```python
from build123d import *

# Parameters (mm, degrees)
BOSS_EXTRUDE1_DEPTH  = 6
CUT_EXTRUDE15_DEPTH  = 103.528044944
SKETCH19_OUTSIDE_W   = 185.536
SKETCH19_OUTSIDE_H   = 176.439
SKETCH19_OUTSIDE_W_2 = 80
SKETCH19_OUTSIDE_H_2 = 40
CUT_EXTRUDE16_DEPTH  = 103.528044944
SKETCH20_R           = 2.4
CUT_EXTRUDE17_DEPTH  = 84.234608187


with BuildPart() as part:
    # Sketch1 → Boss-Extrude1 (new, symmetric)
    with BuildSketch(Plane(origin=(0, 0, 0), x_dir=(1, 0, 0), z_dir=(0, 1, 0))):
        with BuildLine():
            ThreePointArc((36.224522061, -62.223661106), (0, 72), (-36.224522061, -62.223661106))
            ThreePointArc((-36.224522061, -62.223661106), (-32.797800029, -62.818856853), (-29.811944095, -61.035223988))
            ThreePointArc((-29.811944095, -61.035223988), (0, -46.75), (29.811944095, -61.035223988))
            ThreePointArc((29.811944095, -61.035223988), (32.797800029, -62.818856853), (36.224522061, -62.223661106))
        make_face()
    extrude(amount=BOSS_EXTRUDE1_DEPTH, both=True)

    # Sketch17 → Cut-Extrude15 (cut, through all)
    with BuildSketch(Plane(origin=(0, 6, 0), x_dir=(1, 0, 0), z_dir=(0, 1, 0))):
        with BuildLine():
            Line((11.501290376, 48.2), (-11.501290376, 48.2))
            ThreePointArc((-11.501290376, 48.2), (-13.503335986, 55.621683574), (-18.824890953, 61.168811339))
            ThreePointArc((-18.824890953, 61.168811339), (-13.394450398, 62.582654933), (-7.861037919, 63.515384615))
            ThreePointArc((-7.861037919, 63.515384615), (0, 57), (7.861037919, 63.515384615))
            ThreePointArc((7.861037919, 63.515384615), (13.394450398, 62.582654933), (18.824890953, 61.168811339))
            ThreePointArc((18.824890953, 61.168811339), (13.503335986, 55.621683574), (11.501290376, 48.2))
        make_face()
    extrude(amount=-CUT_EXTRUDE15_DEPTH, mode=Mode.SUBTRACT)

    # Sketch19 outside → Cut-Extrude16 (cut, through all)
    with BuildSketch(Plane(origin=(0, 6, 0), x_dir=(1, 0, 0), z_dir=(0, 1, 0))):
        with Locations((0, 4.5485)):
            Rectangle(SKETCH19_OUTSIDE_W, SKETCH19_OUTSIDE_H)
        with Locations((0, 57)):
            Rectangle(SKETCH19_OUTSIDE_W_2, SKETCH19_OUTSIDE_H_2, mode=Mode.SUBTRACT)
    extrude(amount=-CUT_EXTRUDE16_DEPTH, mode=Mode.SUBTRACT)

    # Sketch20 → Cut-Extrude17 (cut, through all)
    with BuildSketch(Plane(origin=(0, 6, 0), x_dir=(1, 0, 0), z_dir=(0, 1, 0))):
        with Locations(Location((0, 65, 0), (0, 0, 270))):
            Circle(SKETCH20_R)
        with Locations(Location((0, 43, 0), (0, 0, 270))):
            Circle(SKETCH20_R)
    extrude(amount=-CUT_EXTRUDE17_DEPTH, mode=Mode.SUBTRACT)


solid = part.part
```
The model under review builds one solid part; all positions refer to its coordinate system, in mm. A direction names the side the tool comes from. Coordinates: 2 decimals unless noted, no trailing zeros. Write each loop counter-clockwise with the first axis right and the second up, starting at its lowest first coordinate (ties: lowest second). Pieces come first, ordered by that corner, then holes. Notation, with made-up numbers: (88, 46) - (95, 46) arc R28 cw to (95, 68) - close; hole circle Ø1 at (15, 76.5). An arc over 180 degrees is marked (long way). Answer in a Markdown table with one row per item. Add a question column.
Q1. Consider section D-D on x = 15.5. Give the boundary of the cut face in (y, z).
Q2. Consider section C-C on z = -43. Give the boundary of the cut face in (x, y).
Q3. Consider section B-B on y = 2. Give the boundary of the cut face in (x, z).
Q4. Clearance check with flat-ended pins moving along their axes: pin 1 (2 mm diameter, centred on x = -32, y = 2.5, fed in from -Z); pin 2 (3 mm diameter, centred on x = 13.5, y = -2.5, fed in from -Z). State where each tip first meets the part, or that it passes through.
Q5. Consider section A-A on x = 0. Give the boundary of the cut face in (y, z).
Q6. For faces 1 (the face through (40, 0, -48)), 2 (the face through (0, 0, -48.2)), list the 3-axis set-ups (+Z, -Z, +X, -X, +Y, -Y) from which the entire face can be reached by the end or side of a thin tool; tool diameter is ignored.
Q7. Draft analysis for pull direction X (two halves, no side actions). For faces 3 (the face through (-13.45, 0.08, -55.53)), 4 (the face through (0.106, 0.084, -45.398)), 5 (the face through (-1, 0, -37)), 6 (the face through (-40, 0, -48)), state which applies: +X half, -X half, draft (parallel to the pull), parting line (faces both ways), or undercut.
Q8. To check wall thickness, follow line 1 along X through (y, z) = (1.5, -43); line 2 along Z through (x, y) = (1, -1.25); line 3 along X through (y, z) = (1.75, -53). State the ranges of each line that lie inside material, in increasing order. Write a range as from..to.
Answers below:
| question | item | result |
|---|---|---|
| 1 | outline | (-6, -70.31) - (6, -70.31) - (6, -62.09) - (-6, -62.09) - close; (-6, -58.39) - (6, -58.39) - (6, -37) - (-6, -37) - close |
| 2 | outline | (-40, -6) - (-2.4, -6) - (-2.4, 6) - (-40, 6) - close; (2.4, -6) - (40, -6) - (40, 6) - (2.4, 6) - close |
| 3 | outline | (-40, -59.87) arc R72 ccw to (40, -59.87) - (40, -37) - (-40, -37) - close; hole (-18.82, -61.17) arc R64 ccw to (-7.86, -63.52) arc R8 cw to (7.86, -63.52) arc R64 ccw to (18.82, -61.17) arc R15.5 cw to (11.5, -48.2) - (-11.5, -48.2) arc R15.5 cw to start; hole circle Ø4.8 at (0, -65); hole circle Ø4.8 at (0, -43) |
| 4 | pin 1 | z = -64.98 |
| 4 | pin 2 | z = -70.99 |
| 5 | outline | (-6, -72) - (6, -72) - (6, -67.4) - (-6, -67.4) - close; (-6, -62.6) - (6, -62.6) - (6, -57) - (-6, -57) - close; (-6, -48.2) - (6, -48.2) - (6, -45.4) - (-6, -45.4) - close; (-6, -40.6) - (6, -40.6) - (6, -37) - (-6, -37) - close |
| 6 | face 1 | +Z, -Z, +X, +Y, -Y |
| 6 | face 2 | +Y, -Y |
| 7 | face 3 | undercut |
| 7 | face 4 | undercut |
| 7 | face 5 | draft |
| 7 | face 6 | -X half |
| 8 | line 1 | -40..-2.4, 2.4..40 |
| 8 | line 2 | -71.99..-67.18, -62.82..-57.06, -48.2..-45.18, -40.82..-37 |
| 8 | line 3 | -40..-12.33, 12.33..40 |
